For this review, take the finished solid that the model builds, in its own axes (mm). Face numbers are marked on the shaded views. A direction names the side the tool comes from. Round coordinates to 2 decimals unless told otherwise and drop trailing zeros. Order: outer loops, then holes, each group sorted by start corner. A loop starts at its lowest first (then second) coordinate and runs counter-clockwise, first axis right, second up. Notation, with made-up numbers: M -9,-9 L 28,-9 A17 cw 28,16 Z; hole C 85.5,73.25 d11. An arc over 180 degrees is marked long. Answer as a JSON object with one key per item and string values.
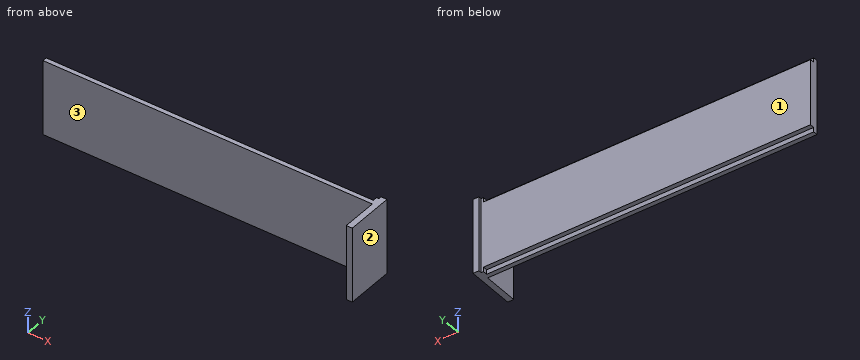
Autodesk Inventor part; units mm, degrees
ref_plane "YZ Plane" through (0, 0, 0) normal (1, 0, 0) x (0, 1, 0)
ref_plane "XZ Plane" through (0, 0, 0) normal (0, 1, 0) x (-1, 0, 0)
ref_plane "XY Plane" through (0, 0, 0) normal (0, 0, 1) x (1, 0, 0)
sketch "Sketch2" plane through (0, 0, 0) normal (0, 1, 0) x (-1, 0, 0)
  line L0 (56, 11) -> (-56, 11)
  line L1 (-56, 11) -> (-56, -11)
  line L2 (-56, -11) -> (56, -11)
  line L3 (56, -11) -> (56, 11)
  line L4 (56, 11) -> (-56, -11) construction
  line L5 (-56, 11) -> (56, -11) construction
  point P0 (0, 0)
  dimension "d2" = 112
  dimension "d3" = 22
extrude "Extrusion1" add sketch "Sketch2" along normal blind 3
sketch "Sketch4" plane through (-56, 0, 11) normal (0, 0, 1) x (1, 0, 0)
  line L0 (0, 0) -> (112, 0)
  line L1 (112, 0) -> (112, 3)
  line L2 (0, 0) -> (110, 0)
  line L3 (112, 0) -> (112, 1.5) construction
  line L4 (112, 1.5) -> (109.25, 1.5) construction
  line L5 (0, 1.5) -> (0, 0)
  line L6 (109.25, 1.5) -> (0, 1.5)
  line L7 (110, 0) -> (112, 0) construction
  line L8 (109.25, 1.5) -> (109.25, 3)
  line L9 (0, 3) -> (112, 3)
  line L10 (109.25, 3) -> (112, 3)
  line L11 (112, 3) -> (112, 0)
  line L12 (110, 0) -> (112, 0)
  point P0 (56, 0)
  dimension "d6" = 1.5
  dimension "d12" = 2.75
extrude "Extrusion2" add sketch "Sketch4" along normal blind 1.5
mirror "Mirror1" about plane through (0, 0, 0) normal (0, 0, 1) of "Extrusion2"
sketch "Sketch6" plane through (0, 0, 0) normal (0, -1, 0) x (1, 0, 0)
  line L0 (56, 12.5) -> (53.25, 12.5)
  line L1 (-56, -12.5) -> (56, -12.5)
  line L2 (56, 12.5) -> (54, 12.5)
  line L3 (54, 12.5) -> (54, -12.5)
  line L4 (54, -12.5) -> (56, -12.5)
  line L5 (56, -12.5) -> (56, 12.5)
  point P0 (0, 0)
  dimension "d13" = 2
extrude "Extrusion4" add sketch "Sketch6" along normal blind 12 and the other way blind 4
properties part number "LampeSolaire2_Casing_Cover"
1) For L1, parallel to X at y = -4, z = 1.5; L2, parallel to Y at x = -20, z = 0.75; L3, parallel to Z at x = -4, y = 2.75, list the stretches that pass through material, from the lowest coordinate up.
Geometry check:
{"L1": "x = 54 to 56", "L2": "y = 0 to 3", "L3": "z = -11 to 11"}
2) Add section C-C on y = -1.25. State the section outline as (x, z) points.
Geometry check:
{"outline": "M 54,-12.5 L 56,-12.5 L 56,12.5 L 54,12.5 Z"}
3) Machinability: for the marked faces 1, 2 and 3, which of the approach directions +Z, -Z, +X, -X, +Y, -Y give a long, thin tool a straight path to every point of the face, cutting with its end or side? Answer none if there is none.
Geometry check:
{"face 1": "+Z, -Z, -X, +Y", "face 2": "+Z, -Z, +X, +Y, -Y", "face 3": "+Z, -Z, -X, -Y"}
4) Insertion check: P1, Ø1.2, axis at x = -9.5, y = 2.5, coming from the -Z side; P2, Ø12, axis at x = -14.5, z = 0, coming from the +Y side; P3, Ø6, axis at y = -6.5, z = 0, coming from the -X side. Each pin has a flat end and moves straight along its axis. Give the tip position at first contact, or say it passes through.
Geometry check:
{"P1": "stops at z = -11", "P2": "stops at y = 3", "P3": "stops at x = 54"}
5) Add section A-A on z = 9. State the section outline as (x, y) points, and give its area (3 significant figures).
Geometry check:
{"outline": "M -56,0 L 54,0 L 54,-12 L 56,-12 L 56,4 L 54,4 L 54,3 L -56,3 Z", "area": "362 mm²"}
6) Add section B-B on x = -7.5. State the section outline as (y, z) points.
Geometry check:
{"outline": "M 0,-12.5 L 1.5,-12.5 L 1.5,-11 L 3,-11 L 3,11 L 1.5,11 L 1.5,12.5 L 0,12.5 Z"}
